```python
from build123d import *

# Parameters (mm, degrees)
SKETCH1_W           = 95.3
SKETCH1_H           = 79
BOSS_EXTRUDE1_DEPTH = 33
SKETCH5_W           = 16.412638375
SKETCH5_H           = 11.424483575
CUT_EXTRUDE3_DEPTH  = 51
SKETCH4_W           = 19.8
SKETCH4_H           = 11.7
CUT_EXTRUDE4_DEPTH  = 51
BOSS_EXTRUDE2_START = 30
BOSS_EXTRUDE2_DEPTH = 3
CUT_EXTRUDE6_START  = 2
SKETCH3_W           = 91.3
SKETCH3_H           = 75
CUT_EXTRUDE6_DEPTH  = 33
BOSS_EXTRUDE3_DEPTH = 33
CUT_EXTRUDE7_START  = 2
CUT_EXTRUDE7_DEPTH  = 33
SKETCH13_W          = 28.277376506
SKETCH13_H          = 18.284619395
CUT_EXTRUDE8_DEPTH  = 63
CUT_EXTRUDE9_START  = 15
SKETCH15_R          = 2.404549827
SKETCH15_R_2        = 2.15
CUT_EXTRUDE9_DEPTH  = 63


with BuildPart() as part:
    # Sketch1 → Boss-Extrude1 (new body)
    with BuildSketch(Plane(origin=(0, 0, 0), x_dir=(1, 0, 0), z_dir=(0, 1, 0))):
        with Locations((1.627011494, 0.770114943)):
            Rectangle(SKETCH1_W, SKETCH1_H)
    extrude(amount=BOSS_EXTRUDE1_DEPTH)

    # Sketch5 → Cut-Extrude3 (cut)
    with BuildSketch(Plane(origin=(0, 0, 0), x_dir=(0, 0, -1), z_dir=(1, 0, 0))):
        with Locations((21.044550583, 16.58045411)):
            Rectangle(SKETCH5_W, SKETCH5_H)
    extrude(amount=CUT_EXTRUDE3_DEPTH, mode=Mode.SUBTRACT)

    # Sketch4 → Cut-Extrude4 (cut)
    with BuildSketch(Plane.XY):
        with Locations((-28.653400332, 16.73218903)):
            Rectangle(SKETCH4_W, SKETCH4_H)
    extrude(amount=CUT_EXTRUDE4_DEPTH, mode=Mode.SUBTRACT)

    # Sketch6 → Boss-Extrude2 (add)
    with BuildSketch(Plane(origin=(0, 0, 0), x_dir=(1, 0, 0), z_dir=(0, 1, 0)).offset(BOSS_EXTRUDE2_START)):
        with BuildLine():
            Line((-54.022988506, -46.729885057), (57.277011494, -46.729885057))
            Line((57.277011494, -46.729885057), (57.277011494, 43.194295461))
            ThreePointArc((57.277011494, 43.194295461), (1.627011494, 48.270114943), (-54.022988506, 43.194295461))
            Line((-54.022988506, 43.194295461), (-54.022988506, -46.729885057))
        make_face()
    extrude(amount=BOSS_EXTRUDE2_DEPTH)

    # Sketch3 → Cut-Extrude6 (cut)
    with BuildSketch(Plane(origin=(0, 0, 0), x_dir=(1, 0, 0), z_dir=(0, 1, 0)).offset(CUT_EXTRUDE6_START)):
        with Locations((1.627011494, 0.770114943)):
            Rectangle(SKETCH3_W, SKETCH3_H)
    extrude(amount=CUT_EXTRUDE6_DEPTH, mode=Mode.SUBTRACT)

    # Sketch7 → Boss-Extrude3 (add)
    with BuildSketch(Plane(origin=(0, 0, 0), x_dir=(1, 0, 0), z_dir=(0, 1, 0))):
        with BuildLine():
            Line((-54.022988506, -46.729885057), (-60.700936328, -53.40783288))
            Line((-60.700936328, -53.40783288), (-96.723977713, -34.253129761))
            Line((-96.723977713, -34.253129761), (-130.872988506, 18.270114943))
            ThreePointArc((-130.872988506, 18.270114943), (1.627011494, 48.270114943), (134.127011494, 18.270114943))
            Line((134.127011494, 18.270114943), (99.978000701, -34.253129761))
            Line((99.978000701, -34.253129761), (63.954959317, -53.40783288))
            Line((63.954959317, -53.40783288), (57.277011494, -46.729885057))
            Line((57.277011494, -46.729885057), (-54.022988506, -46.729885057))
        make_face()
    extrude(amount=BOSS_EXTRUDE3_DEPTH)

    # Sketch12 → Cut-Extrude7 (cut)
    with BuildSketch(Plane(origin=(0, 0, 0), x_dir=(1, 0, 0), z_dir=(0, 1, 0)).offset(CUT_EXTRUDE7_START)):
        with BuildLine():
            Line((-55.675241183, -44.247946624), (-61.717664186, -40.981103814))
            Line((-61.717664186, -40.981103814), (-67.147920345, -47.148292557))
            Line((-67.147920345, -47.148292557), (-94.980050769, -32.348981479))
            Line((-94.980050769, -32.348981479), (-122.582923998, 10.105907593))
            ThreePointArc((-122.582923998, 10.105907593), (-116.666047132, 14.289696558), (-118.009133951, 21.410766685))
            ThreePointArc((-118.009133951, 21.410766685), (1.346034443, 45.347959229), (120.701202837, 21.410766685))
            ThreePointArc((120.701202837, 21.410766685), (119.358116018, 14.289696558), (125.274992883, 10.105907593))
            Line((125.274992883, 10.105907593), (95.518671487, -34.090338294))
            Line((95.518671487, -34.090338294), (69.839989231, -47.148292557))
            Line((69.839989231, -47.148292557), (64.409733071, -40.981103814))
            Line((64.409733071, -40.981103814), (58.367310069, -44.247946624))
            Line((58.367310069, -44.247946624), (-55.675241183, -44.247946624))
        make_face()
    extrude(amount=CUT_EXTRUDE7_DEPTH, mode=Mode.SUBTRACT)

    # Sketch13 → Cut-Extrude8 (cut)
    with BuildSketch(Plane.XY):
        with Locations((2.186144679, 17.976259721)):
            Rectangle(SKETCH13_W, SKETCH13_H)
    extrude(amount=CUT_EXTRUDE8_DEPTH, mode=Mode.SUBTRACT)

    # Sketch15 → Cut-Extrude9 (cut)
    with BuildSketch(Plane(origin=(0, 0, 0), x_dir=(1, 0, 0), z_dir=(0, 1, 0)).offset(CUT_EXTRUDE9_START)):
        with Locations(Location((-122.881880972, 16.804537187, 0), (0, 0, 270))):
            Circle(SKETCH15_R)
        with Locations(Location((-60.728139954, -47.058565961, 0), (0, 0, 270))):
            Circle(SKETCH15_R_2)
        with Locations(Location((63.420208839, -47.058565961, 0), (0, 0, 90))):
            Circle(SKETCH15_R_2)
        with Locations(Location((125.573949857, 16.804537187, 0), (0, 0, 90))):
            Circle(SKETCH15_R)
    extrude(amount=CUT_EXTRUDE9_DEPTH, mode=Mode.SUBTRACT)


solid = part.part
```
The listing builds one solid part. Answer for the finished solid, in the listing's coordinates (mm). A direction names the side the tool comes from. Give positions to 0.01 mm unless a question says otherwise; leave off trailing zeros. Order: outer loops, then holes, each group sorted by start corner. A loop starts at its lowest first (then second) coordinate and runs counter-clockwise, first axis right, second up.
1) Find section C-C on y = 11.5. Write down the section's boundary in (x, z) (3 decimals), then the cut area to 3 significant figures.
Reported:
outline: (-130.873, -18.27) arc R307.604 ccw to (134.127, -18.27) - (99.978, 34.253) - (63.955, 53.408) - (57.277, 46.73) - (16.325, 46.73) - (16.325, 44.248) - (58.367, 44.248) - (64.41, 40.981) - (69.84, 47.148) - (95.519, 34.09) - (125.275, -10.106) arc R6.705 ccw to (120.701, -21.411) arc R309.532 cw to (-118.009, -21.411) arc R6.705 ccw to (-122.583, -10.106) - (-94.98, 32.349) - (-67.148, 47.148) - (-61.718, 40.981) - (-55.675, 44.248) - (-11.953, 44.248) - (-11.953, 46.73) - (-54.023, 46.73) - (-60.701, 53.408) - (-96.724, 34.253) - close
area: 1,820 mm2
2) Given P1, Ø4.5, axis at x = -122.88, z = -16.8, coming from the +Y side; P2, Ø6, axis at y = 14.5, z = -26.5, coming from the +X side; P3, Ø0.7, axis at y = 13.5, z = 45, coming from the +X side, each flat-ended and moving along its own axis, determine where each tip first touches the part or whether it passes through.
Reported:
P1: stops at y = 15
P2: stops at x = 122.56
P3: stops at x = 80.43
3) Find section A-A on y = 23.5. Write down the section's boundary in (x, z) (3 decimals).
Reported:
outline: (-130.873, -18.27) arc R307.604 ccw to (134.127, -18.27) - (99.978, 34.253) - (63.955, 53.408) - (57.277, 46.73) - (16.325, 46.73) - (16.325, 44.248) - (58.367, 44.248) - (64.41, 40.981) - (69.84, 47.148) - (95.519, 34.09) - (125.275, -10.106) arc R6.705 ccw to (120.701, -21.411) arc R309.532 cw to (-118.009, -21.411) arc R6.705 ccw to (-122.583, -10.106) - (-94.98, 32.349) - (-67.148, 47.148) - (-61.718, 40.981) - (-55.675, 44.248) - (-11.953, 44.248) - (-11.953, 46.73) - (-54.023, 46.73) - (-60.701, 53.408) - (-96.724, 34.253) - close; hole circle Ø4.809 at (-122.882, -16.805); hole circle Ø4.3 at (-60.728, 47.059); hole circle Ø4.3 at (63.42, 47.059); hole circle Ø4.809 at (125.574, -16.805)
4) Consider line 1 along Y through (x, z) = (71, 32); line 2 along X through (y, z) = (17, 6); line 3 along Z through (x, y) = (88, 8). Determine where each line is inside the solid, lowest interval first.
Reported:
line 1: y = 0 to 2
line 2: x = -115.09 to -112.11, 114.43 to 118.35
line 3: z = -35.89 to -32.97, 37.91 to 40.62
5) Determine the mould class of faces 1 (the face through (-61, 15, 47)), 2 (the face through (117.292, 16.269, 7.624)), 3 (the face through (3, 0, 2)) for opening direction X: pulls with the +X half, pulls with the -X half, needs draft (parallel to the pull), parting line crosses it, or undercut.
Reported:
face 1: undercut
face 2: pulls with the +X half
face 3: needs draft
6) Find section D-D on x = 31.5. Write down the section's boundary in (y, z), then the cut area to 3 significant figures.
Reported:
outline: (0, -46.82) - (33, -46.82) - (33, -43.88) - (2, -43.88) - (2, 44.25) - (33, 44.25) - (33, 46.73) - (0, 46.73) - close
area: 355 mm2
7) For faces 4 (the face through (60.663, 16.269, 50.116)), 5 (the face through (-113.56, 16.27, 8.36)), 6 (the face through (-58.915, 23.874, 48.214)), determine the directions among +Z, -Z, +X, -X, +Y, -Y from which every point of the face is accessible in a straight line to the end or side of a thin tool.
Reported:
face 4: +Z, +Y, -Y
face 5: +Z, -X, +Y, -Y
face 6: +Y
